Geometry check sheet. Reference: drawing and pictorial views, mm from the part's lowest x, y, z. A direction names the side the tool comes from. Round coordinates to 2 decimals unless told otherwise and drop trailing zeros. Loops run counter-clockwise (first coordinate to the right, second up) from the corner with the lowest first, then second, coordinate; pieces in that order, holes last. Notation, with made-up numbers: (-39, 46.25) -> (-35, 46.25) arc R26 ccw to (-35, 70.25) -> close; hole circle Ø10 at (75, 34.25). An arc over 180 degrees is marked (long way). Write item = value, one per line.
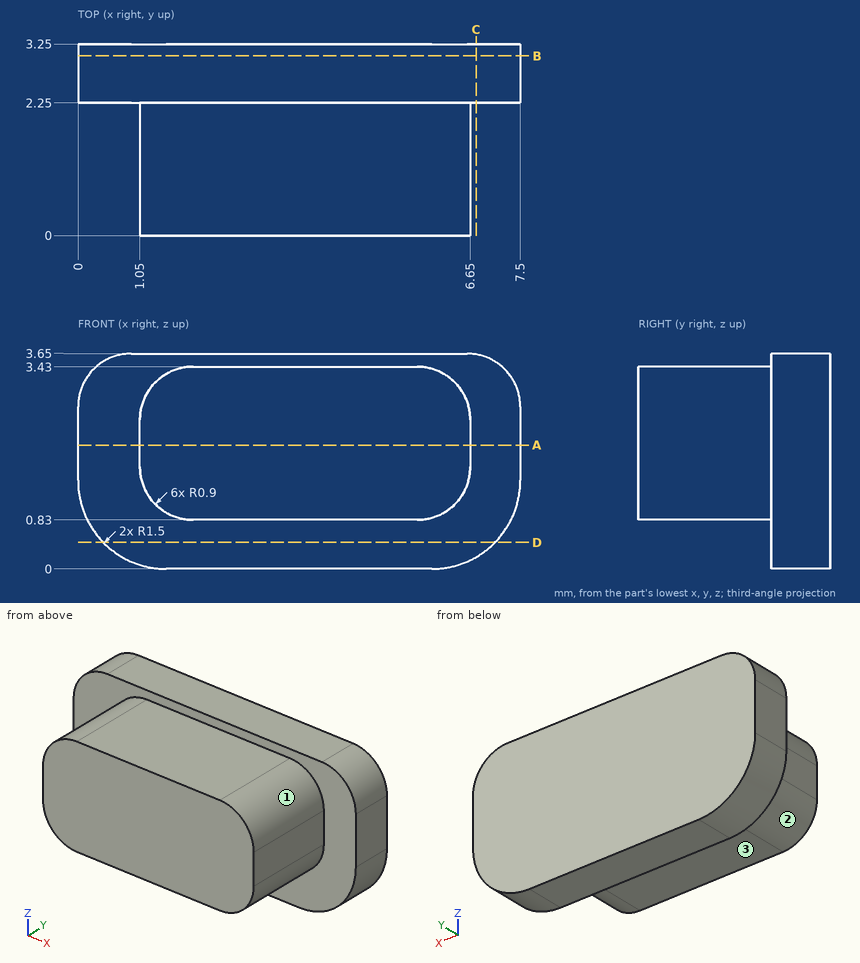
(1) Sectioned sample at A-A, the plane z = 2.1. Record the cut outline in (x, y).
Filled sheet:
outline = (0, 2.25) -> (1.05, 2.25) -> (1.05, 0) -> (6.65, 0) -> (6.65, 2.25) -> (7.5, 2.25) -> (7.5, 3.25) -> (0, 3.25) -> close
(2) Set-up check for the marked faces 1, 2 and 3: record each of +Z, -Z, +X, -X, +Y, -Y from which the full face is reachable in a straight line by a thin tool's end or side.
Filled sheet:
face_1 = +Z, +X, -Y
face_2 = -Z, -X, -Y
face_3 = -Z, +X, -X, -Y
(3) Sectioned sample at C-C, the plane x = 6.75. Record the cut outline in (y, z).
Filled sheet:
outline = (2.25, 0.2) -> (3.25, 0.2) -> (3.25, 3.64) -> (2.25, 3.64) -> close
(4) Sectioned sample at B-B, the plane y = 3.05. Record the cut outline in (x, z), and give its area (3 significant figures).
Filled sheet:
outline = (0, 1.5) arc R1.5 ccw to (1.5, 0) -> (6, 0) arc R1.5 ccw to (7.5, 1.5) -> (7.5, 2.75) arc R0.9 ccw to (6.6, 3.65) -> (0.9, 3.65) arc R0.9 ccw to (0, 2.75) -> close
area = 26.1 mm2
(5) Material ranges on probe 1 along Z at (x, y) = (4.5, 0.7); probe 2 along Y at (x, z) = (2.75, 0.45); probe 3 along X at (y, z) = (1.75, 2.05), recorded low to high. Write a range as from..to.
Filled sheet:
probe_1 = 0.83..3.43
probe_2 = 2.25..3.25
probe_3 = 1.05..6.65
(6) Go/stop test with flat-tipped pins: pin 1 Ø1.5 at (y, z) = (0.5, 2.5) entering from -X; pin 2 Ø1.1 at (x, y) = (3.5, 1.5) entering from +Z; pin 3 Ø0.9 at (y, z) = (1.5, 2.5) entering from +X. Record where each tip stops, or that it passes through.
Filled sheet:
pin_1 = 1.05
pin_2 = 3.43
pin_3 = 6.65
(7) Sectioned sample at D-D, the plane z = 0.45. Record the cut outline in (x, y), and give its area (3 significant figures).
Filled sheet:
outline = (0.43, 2.25) -> (7.07, 2.25) -> (7.07, 3.25) -> (0.43, 3.25) -> close
area = 6.64 mm2
